```python
from build123d import *

# Parameters (mm, degrees)
SALIENTE_EXTRUIR1_DEPTH   = 1
CROQUIS2_R                = 1
CORTAR_EXTRUIR1_DEPTH     = 23.164160259
SIMETR_A2_COPY_1_SKETCH_R = 1
SIMETR_A2_COPY_1_DEPTH    = 23.164160259


with BuildPart() as part:
    # Croquis1 → Saliente-Extruir1 (new body)
    with BuildSketch(Plane(origin=(0, 0, 0), x_dir=(1, 0, 0), z_dir=(0, 1, 0))):
        with BuildLine():
            Line((19, -9.5), (-19, -9.5))
            ThreePointArc((-19, -9.5), (-19.707106781, -9.207106781), (-20, -8.5))
            Line((-20, -8.5), (-20, 8.5))
            ThreePointArc((-20, 8.5), (-19.707106781, 9.207106781), (-19, 9.5))
            Line((-19, 9.5), (19, 9.5))
            ThreePointArc((19, 9.5), (19.707106781, 9.207106781), (20, 8.5))
            Line((20, 8.5), (20, -8.5))
            ThreePointArc((20, -8.5), (19.707106781, -9.207106781), (19, -9.5))
        make_face()
    extrude(amount=SALIENTE_EXTRUIR1_DEPTH)

    # Croquis2 → Cortar-Extruir1 (cut, through all)
    with BuildSketch(Plane.XZ):
        with Locations(Location((17, 6.5, 0), (0, 0, 270))):
            Circle(CROQUIS2_R)
    cortar_extruir1 = extrude(amount=-CORTAR_EXTRUIR1_DEPTH, mode=Mode.SUBTRACT)

    # Simetr_a1: Cortar-Extruir1 across plane
    add(cortar_extruir1.mirror(Plane(origin=(0, 0, 0), x_dir=(1, 0, 0), z_dir=(0, 0, -1))), mode=Mode.SUBTRACT)

    # Simetr_a2: Cortar-Extruir1 across plane
    add(cortar_extruir1.mirror(Plane(origin=(0, 0, 0), x_dir=(0, 0, 1), z_dir=(1, 0, 0))), mode=Mode.SUBTRACT)

    # Simetr_a2 copy 1 sketch → Simetr_a2 copy 1 (cut, through all)
    with BuildSketch(Plane(origin=(0, 0, 0), x_dir=(-1, 0, 0), z_dir=(0, -1, 0))):
        with Locations(Location((17, 6.5, 0), (0, 0, 270))):
            Circle(SIMETR_A2_COPY_1_SKETCH_R)
    extrude(amount=-SIMETR_A2_COPY_1_DEPTH, mode=Mode.SUBTRACT)


solid = part.part
```
Could you check a few things on this model? Use its own coordinates, in mm. Round coordinates to 2 decimals unless told otherwise and drop trailing zeros. Loops run counter-clockwise (first coordinate to the right, second up) from the corner with the lowest first, then second, coordinate; pieces in that order, holes last. Notation, with made-up numbers: (21, 29) -> (74, 29) arc R9 cw to (74, 41) -> close; hole circle Ø6 at (-8, 63). An arc over 180 degrees is marked (long way). One line per question, with ' | ' between items.
(1) If we section it at C-C on y = 0.2: List the corners of the cut face in (x, z) for me, and give its area (3 significant figures).
Model answer:
outline: (-20, -8.5) arc R1 ccw to (-19, -9.5) -> (19, -9.5) arc R1 ccw to (20, -8.5) -> (20, 8.5) arc R1 ccw to (19, 9.5) -> (-19, 9.5) arc R1 ccw to (-20, 8.5) -> close; hole circle Ø2 at (-17, -6.5); hole circle Ø2 at (-17, 6.5); hole circle Ø2 at (17, -6.5); hole circle Ø2 at (17, 6.5) | area: 747 mm^2
(2) If we section it at A-A on x = 17: List the corners of the cut face in (y, z) for me, and give its area (3 significant figures).
Model answer:
outline: (0, -9.5) -> (1, -9.5) -> (1, -7.5) -> (0, -7.5) -> close; (0, -5.5) -> (1, -5.5) -> (1, 5.5) -> (0, 5.5) -> close; (0, 7.5) -> (1, 7.5) -> (1, 9.5) -> (0, 9.5) -> close | area: 15.0 mm^2
(3) If I drill on probe 1 along X at (y, z) = (0.7, 6.5); probe 2 along Z at (x, y) = (-17, 0.2), over which ranges is the centre line in solid material (lowest first)?
Model answer:
probe 1: x = -20 to -18, -16 to 16, 18 to 20 | probe 2: z = -9.5 to -7.5, -5.5 to 5.5, 7.5 to 9.5
(4) Thinking about a two-plate mould opening in Z: for faces 1 (the face through (16.024, 0.493, 6.717)), 2 (the face through (16.024, 0.493, -6.717)), 3 (the face through (-20, 0.5, 0.1)), 4 (the face through (-0.3, 0.5, -9.5)), which applies, released by +Z, released by -Z, zero draft, split by the parting line, or undercut?
Model answer:
face 1: undercut | face 2: undercut | face 3: zero draft | face 4: released by -Z
(5) If we section it at B-B on z = -6.5: List the corners of the cut face in (x, y) for me.
Model answer:
outline: (-20, 0) -> (-18, 0) -> (-18, 1) -> (-20, 1) -> close; (-16, 0) -> (16, 0) -> (16, 1) -> (-16, 1) -> close; (18, 0) -> (20, 0) -> (20, 1) -> (18, 1) -> close
